Geometry: final body of the model. Coordinates: model frame, mm. Face numbers are marked on the shaded views. A direction names the side the tool comes from. Give positions to 0.01 mm unless a question says otherwise; leave off trailing zeros. Write each loop counter-clockwise with the first axis right and the second up, starting at its lowest first coordinate (ties: lowest second). Pieces come first, ordered by that corner, then holes. Notation, with made-up numbers: (62, 79) -> (103, 79) arc R23 cw to (103, 110) -> close; hole circle Ø10 at (19.5, 32.5). An arc over 180 degrees is marked (long way). Use CSV: the item, a comma, the result in double quotes. Start each with the question number.
1) Material intervals for line 1 (Z direction, x = -3, y = -1); line 2 (Y direction, x = -2.5, z = -0.8); line 3 (Y direction, x = -10, z = -0.7), sorted ascending. Write a range as [from, to].
2) Section B-B (x = 8). Output: boundary loops of the cut face in (y, z).
3) Section D-D (z = -2.6). Output: boundary loops of the cut face in (x, y).
4) Section A-A (y = 0). Output: boundary loops of the cut face in (x, z).
5) Section C-C (z = -0.9). Count the separate pieces of the cut face and the enclosed holes in it, plus the area to 3 significant figures.
6) Draft query along Y for the marked faces 1, 2, 3 and 4. Return one class per face: pulls with the +Y half, pulls with the -Y half, needs draft (parallel to the pull), parting line crosses it, or undercut.
7) Set-up query: the marked faces 5 and 6. Return all of +Z, -Z, +X, -X, +Y, -Y with unobstructed straight access to the full face (end or side cutting, diameter ignored); none if empty.
8) Contact query for flat-ended pins moving along their axis: P1, Ø0.6, axis at y = 4.5, z = -1, coming from the +X side; P2, Ø1, axis at y = -5.5, z = -0.5, coming from the +X side; P3, Ø1, axis at y = 0, z = -1, coming from the -X side; P4, Ø1.4, axis at y = -5.5, z = -0.5, coming from the -X side. Output: stop coordinate, or through.
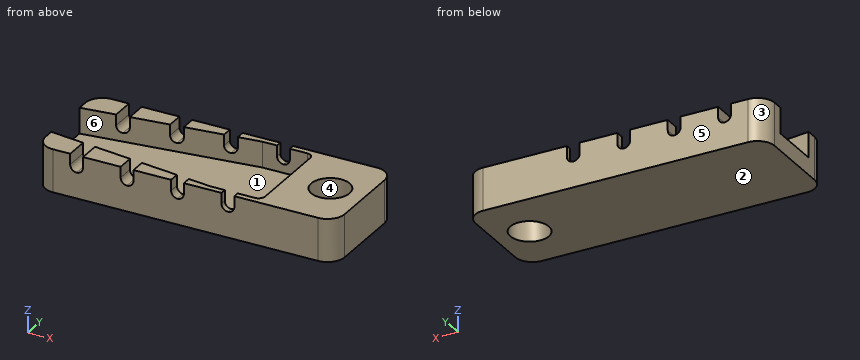
```python
from build123d import *

# Parameters (mm, degrees)
F0_W     = 1.5
F0_H     = 0.7
F0_R     = 2.25
F0_H_2   = 11.1
F0_W_2   = 2.8
F1_DEPTH = 5
F2_DEPTH = 3
F3_DEPTH = 2
F4_R     = 0.74999
F5_R     = 2


# Not quite as in the source:
# - a fillet or chamfer is up to 0.001 mm smaller than in the source, because OpenCascade refuses the exact size


with BuildPart() as f1:
    # F0 (on Top) → F1 (new body)
    with BuildSketch(Plane.XY):
        Polygon((-18.8879279066, 6.25), (-22.8879279066, 6.25), (-22.8879279066, 3), (-18.8879279066, 3.51), align=None)
        Polygon((-17.3879279066, 6.25), (-18.8879279066, 6.25), (-18.8879279066, 3.51), (-17.3879279066, 3.70125), align=None)
        Polygon((-18.8879279066, 3.51), (-22.8879279066, 3), (-22.8879279066, -3), (-18.8879279066, -3.51), align=None)
        Polygon((-12.9879279066, 6.25), (-17.3879279066, 6.25), (-17.3879279066, 3.70125), (-12.9879279066, 4.26225), align=None)
        Polygon((-18.8879279066, -3.51), (-22.8879279066, -3), (-22.8879279066, -6.25), (-18.8879279066, -6.25), align=None)
        Polygon((-11.4879279066, 6.25), (-12.9879279066, 6.25), (-12.9879279066, 4.26225), (-11.4879279066, 4.4535), align=None)
        Polygon((-17.3879279066, -3.70125), (-18.8879279066, -3.51), (-18.8879279066, -6.25), (-17.3879279066, -6.25), align=None)
        Polygon((-7.0879279066, 6.25), (-11.4879279066, 6.25), (-11.4879279066, 4.4535), (-7.0879279066, 5.0145), align=None)
        Polygon((-12.9879279066, -4.26225), (-17.3879279066, -3.70125), (-17.3879279066, -6.25), (-12.9879279066, -6.25), align=None)
        Polygon((-5.5879279066, 6.25), (-7.0879279066, 6.25), (-7.0879279066, 5.0145), (-5.5879279066, 5.20575), align=None)
        Polygon((-11.4879279066, -4.4535), (-12.9879279066, -4.26225), (-12.9879279066, -6.25), (-11.4879279066, -6.25), align=None)
        Polygon((-1.1879279066, 6.25), (-5.5879279066, 6.25), (-5.5879279066, 5.20575), (-2.8879279066, 5.55), (-1.1879279066, 5.55), align=None)
        Polygon((-7.0879279066, -5.0145), (-11.4879279066, -4.4535), (-11.4879279066, -6.25), (-7.0879279066, -6.25), align=None)
        with Locations((-0.4379279066, 5.9)):
            Rectangle(F0_W, F0_H)
        Polygon((-5.5879279066, -5.20575), (-7.0879279066, -5.0145), (-7.0879279066, -6.25), (-5.5879279066, -6.25), align=None)
        Polygon((12.1120720934, 6.25), (0.3120720934, 6.25), (0.3120720934, 5.55), (3.1120720934, 5.55), (3.1120720934, -5.55), (0.3120720934, -5.55), (0.3120720934, -6.25), (12.1120720934, -6.25), align=None)
        with Locations((8.1120720934, 0)):
            Circle(F0_R, mode=Mode.SUBTRACT)
        Polygon((-2.8879279066, -5.55), (-5.5879279066, -5.20575), (-5.5879279066, -6.25), (-1.1879279066, -6.25), (-1.1879279066, -5.55), align=None)
        with Locations((-0.4379279066, -5.9)):
            Rectangle(F0_W, F0_H)
        with Locations((-0.4379279066, 0)):
            Rectangle(F0_W, F0_H_2)
        Polygon((-5.5879279066, 5.20575), (-7.0879279066, 5.0145), (-7.0879279066, -5.0145), (-5.5879279066, -5.20575), align=None)
        Polygon((-17.3879279066, 3.70125), (-18.8879279066, 3.51), (-18.8879279066, -3.51), (-17.3879279066, -3.70125), align=None)
        Polygon((-12.9879279066, 4.26225), (-17.3879279066, 3.70125), (-17.3879279066, -3.70125), (-12.9879279066, -4.26225), align=None)
        Polygon((-7.0879279066, 5.0145), (-11.4879279066, 4.4535), (-11.4879279066, -4.4535), (-7.0879279066, -5.0145), align=None)
        Polygon((-11.4879279066, 4.4535), (-12.9879279066, 4.26225), (-12.9879279066, -4.26225), (-11.4879279066, -4.4535), align=None)
        Polygon((-2.8879279066, 5.55), (-5.5879279066, 5.20575), (-5.5879279066, -5.20575), (-2.8879279066, -5.55), (-1.1879279066, -5.55), (-1.1879279066, 5.55), align=None)
        with Locations((1.7120720934, 0)):
            Rectangle(F0_W_2, F0_H_2)
    extrude(amount=-F1_DEPTH)

    # F0 (on Top) → F2 (cut)
    with BuildSketch(Plane.XY):
        Polygon((-18.8879279066, 3.51), (-22.8879279066, 3), (-22.8879279066, -3), (-18.8879279066, -3.51), align=None)
        Polygon((-17.3879279066, 3.70125), (-18.8879279066, 3.51), (-18.8879279066, -3.51), (-17.3879279066, -3.70125), align=None)
        Polygon((-12.9879279066, 4.26225), (-17.3879279066, 3.70125), (-17.3879279066, -3.70125), (-12.9879279066, -4.26225), align=None)
        Polygon((-11.4879279066, 4.4535), (-12.9879279066, 4.26225), (-12.9879279066, -4.26225), (-11.4879279066, -4.4535), align=None)
        Polygon((-7.0879279066, 5.0145), (-11.4879279066, 4.4535), (-11.4879279066, -4.4535), (-7.0879279066, -5.0145), align=None)
        Polygon((-5.5879279066, 5.20575), (-7.0879279066, 5.0145), (-7.0879279066, -5.0145), (-5.5879279066, -5.20575), align=None)
        Polygon((-2.8879279066, 5.55), (-5.5879279066, 5.20575), (-5.5879279066, -5.20575), (-2.8879279066, -5.55), (-1.1879279066, -5.55), (-1.1879279066, 5.55), align=None)
        with Locations((-0.4379279066, 0)):
            Rectangle(F0_W, F0_H_2)
        with Locations((1.7120720934, 0)):
            Rectangle(F0_W_2, F0_H_2)
    extrude(amount=-F2_DEPTH, mode=Mode.SUBTRACT)

    # F0 (on Top) → F3 (cut)
    with BuildSketch(Plane.XY):
        Polygon((-17.3879279066, 6.25), (-18.8879279066, 6.25), (-18.8879279066, 3.51), (-17.3879279066, 3.70125), align=None)
        Polygon((-11.4879279066, 6.25), (-12.9879279066, 6.25), (-12.9879279066, 4.26225), (-11.4879279066, 4.4535), align=None)
        Polygon((-5.5879279066, 6.25), (-7.0879279066, 6.25), (-7.0879279066, 5.0145), (-5.5879279066, 5.20575), align=None)
        with Locations((-0.4379279066, -5.9)):
            Rectangle(F0_W, F0_H)
        Polygon((-17.3879279066, -3.70125), (-18.8879279066, -3.51), (-18.8879279066, -6.25), (-17.3879279066, -6.25), align=None)
        Polygon((-11.4879279066, -4.4535), (-12.9879279066, -4.26225), (-12.9879279066, -6.25), (-11.4879279066, -6.25), align=None)
        Polygon((-5.5879279066, -5.20575), (-7.0879279066, -5.0145), (-7.0879279066, -6.25), (-5.5879279066, -6.25), align=None)
        with Locations((-0.4379279066, 5.9)):
            Rectangle(F0_W, F0_H)
    extrude(amount=-F3_DEPTH, mode=Mode.SUBTRACT)

    # F4 (radius 0.75 in the source; OpenCascade refuses exactly that, so slightly less here)
    f4_edges = [f1.edges().sort_by_distance(p)[0] for p in [
        (-17.387928, -4.975625, -2),
        (-11.487928, -5.35175, -2),
        (-5.587928, -5.727875, -2),
        (0.312072, -5.9, -2),
        (-18.887928, -4.88, -2),
        (-12.987928, -5.256125, -2),
        (-7.087928, -5.63225, -2),
        (-1.187928, -5.9, -2),
        (-18.887928, 4.88, -2),
        (-12.987928, 5.256125, -2),
        (-7.087928, 5.63225, -2),
        (-1.187928, 5.9, -2),
        (-17.387928, 4.975625, -2),
        (-11.487928, 5.35175, -2),
        (-5.587928, 5.727875, -2),
        (0.312072, 5.9, -2),
        (3.112072, 5.55, -1.5),
        (3.112072, -5.55, -1.5),
    ]]
    fillet(f4_edges, radius=F4_R)

    # F5
    f5_edges = [f1.edges().sort_by_distance(p)[0] for p in [
        (-22.887928, -6.25, -2.5),
        (-22.887928, 6.25, -2.5),
        (12.112072, -6.25, -2.5),
        (12.112072, 6.25, -2.5),
    ]]
    fillet(f5_edges, radius=F5_R)


solid = f1.part
```
Answers follow:
1,line 1,"z = [-5, -3]"
1,line 2,"y = [-6.25, -5.55], [5.55, 6.25]"
1,line 3,"y = [-6.25, -4.64], [4.64, 6.25]"
2,outline,"(-6.25, -5) -> (-2.25, -5) -> (-2.25, 0) -> (-6.25, 0) -> close; (2.25, -5) -> (6.25, -5) -> (6.25, 0) -> (2.25, 0) -> close"
3,outline,"(-22.89, -4.25) arc R2 ccw to (-20.89, -6.25) -> (10.11, -6.25) arc R2 ccw to (12.11, -4.25) -> (12.11, 4.25) arc R2 ccw to (10.11, 6.25) -> (-20.89, 6.25) arc R2 ccw to (-22.89, 4.25) -> (-22.89, 3) -> (-2.89, 5.55) -> (2.36, 5.55) arc R0.75 cw to (3.11, 4.8) -> (3.11, -4.8) arc R0.75 cw to (2.36, -5.55) -> (-2.89, -5.55) -> (-22.89, -3) -> close; hole circle Ø4.5 at (8.11, 0)"
4,outline,"(-22.89, -5) -> (5.86, -5) -> (5.86, 0) -> (3.11, 0) -> (3.11, -3) -> (-22.89, -3) -> close; (10.36, -5) -> (12.11, -5) -> (12.11, 0) -> (10.36, 0) -> close"
5,separate pieces,"9"
5,enclosed holes,"1"
5,area,"162 mm^2"
6,face 1,"undercut"
6,face 2,"needs draft"
6,face 3,"pulls with the +Y half"
6,face 4,"undercut"
7,face 5,"+Z, -Z, +X, -X, +Y"
7,face 6,"+Z"
8,P1,"stops at x = 12.11"
8,P2,"stops at x = 11.97"
8,P3,"stops at x = 3.11"
8,P4,"stops at x = -22.81"
